The listing builds one solid part. Answer for the finished solid, in the listing's coordinates (mm). Give positions to 0.01 mm unless a question says otherwise; leave off trailing zeros. Loops run counter-clockwise (first coordinate to the right, second up) from the corner with the lowest first, then second, coordinate; pieces in that order, holes last. Notation, with made-up numbers: (74, 57.5) - (100, 57.5) arc R25 cw to (100, 89.5) - close; hole circle Ø11 at (56.25, -38). An arc over 180 degrees is marked (long way). Answer as CSV lines item,"result". Start each with the question number.
1) A cutting plane is placed at D-D (x = 7.5). Determine the outline of the cut face in (y, z).
2) A cutting plane is placed at B-B (x = 1.75). Determine the outline of the cut face in (y, z).
3) A cutting plane is placed at A-A (z = 8). Determine the outline of the cut face in (x, y).
4) A cutting plane is placed at C-C (y = 4.2). Determine the outline of the cut face in (x, z), and give its area (3 significant figures).
5) Find the intervals of material crossed by line 1 along Z through (x, y) = (17, 4.9); line 2 along Y through (x, z) = (18.75, 32); line 3 along Z through (x, y) = (18, 3.4), in increasing order.
6) Flat-ended cylindrical pins translate along their axes: pin 1 (6 mm diameter, centred on x = -1, z = 9, fed in from -Y); pin 2 (1.8 mm diameter, centred on x = -6, z = 8, fed in from -Y); pin 3 (3.5 mm diameter, centred on x = 13.5, y = 2, fed in from +Z). Find the tip coordinate at first contact, or state that the pin passes through.
```python
from build123d import *

# Parameters (mm, degrees)
F1_DEPTH = 2
F2_DEPTH = 50
F3_R     = 1.5
F4_DEPTH = 25
F5_R     = 3


with BuildPart() as f1:
    # F0 (on Top) → F1 (new body)
    with BuildSketch(Plane.XY):
        Polygon((3, 3), (0, 0), (18, 0), (15, 3), align=None)
    extrude(amount=F1_DEPTH)

    # F0 (on Top) → F2 (join)
    with BuildSketch(Plane.XY):
        Polygon((-9, 3), (3, 3), (15, 3), (20, 3), (20, 6), (-9, 6), align=None)
    extrude(amount=F2_DEPTH)

    # F3 (on face) → F4 (cut)
    with BuildSketch(Plane(origin=(0, 6, 0), x_dir=(-1, 0, 0), z_dir=(0, 1, 0))):
        with Locations((6, 8)):
            Circle(F3_R)
        with Locations((-17, 8)):
            Circle(F3_R)
        with Locations((-17, 47)):
            Circle(F3_R)
        with Locations((6, 47)):
            Circle(F3_R)
    extrude(amount=-F4_DEPTH, mode=Mode.SUBTRACT)

    # F5
    f5_edges = [f1.edges().sort_by_distance(p)[0] for p in [
        (-9, 4.5, 50),
        (20, 4.5, 50),
    ]]
    fillet(f5_edges, radius=F5_R)


solid = f1.part
```
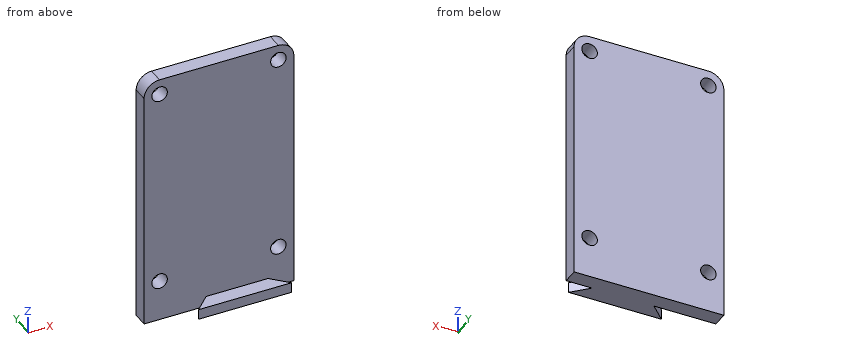
Ans:
1,outline,"(0, 0) - (6, 0) - (6, 50) - (3, 50) - (3, 2) - (0, 2) - close"
2,outline,"(0, 0) - (1.75, 0) - (1.75, 2) - (0, 2) - close; (3, 0) - (6, 0) - (6, 50) - (3, 50) - close"
3,outline,"(-9, 3) - (-7.5, 3) - (-7.5, 6) - (-9, 6) - close; (-4.5, 3) - (15.5, 3) - (15.5, 6) - (-4.5, 6) - close; (18.5, 3) - (20, 3) - (20, 6) - (18.5, 6) - close"
4,outline,"(-9, 0) - (20, 0) - (20, 47) arc R3 ccw to (17, 50) - (-6, 50) arc R3 ccw to (-9, 47) - close; hole circle Ø3 at (-6, 8); hole circle Ø3 at (-6, 47); hole circle Ø3 at (17, 8); hole circle Ø3 at (17, 47)"
4,area,"1,420 mm2"
5,line 1,"0 to 6.5, 9.5 to 45.5, 48.5 to 50"
5,line 2,"3 to 6"
5,line 3,"0 to 6.88, 9.12 to 45.88, 48.12 to 49.83"
6,pin 1,"y = 3"
6,pin 2,"through"
6,pin 3,"z = 50"
